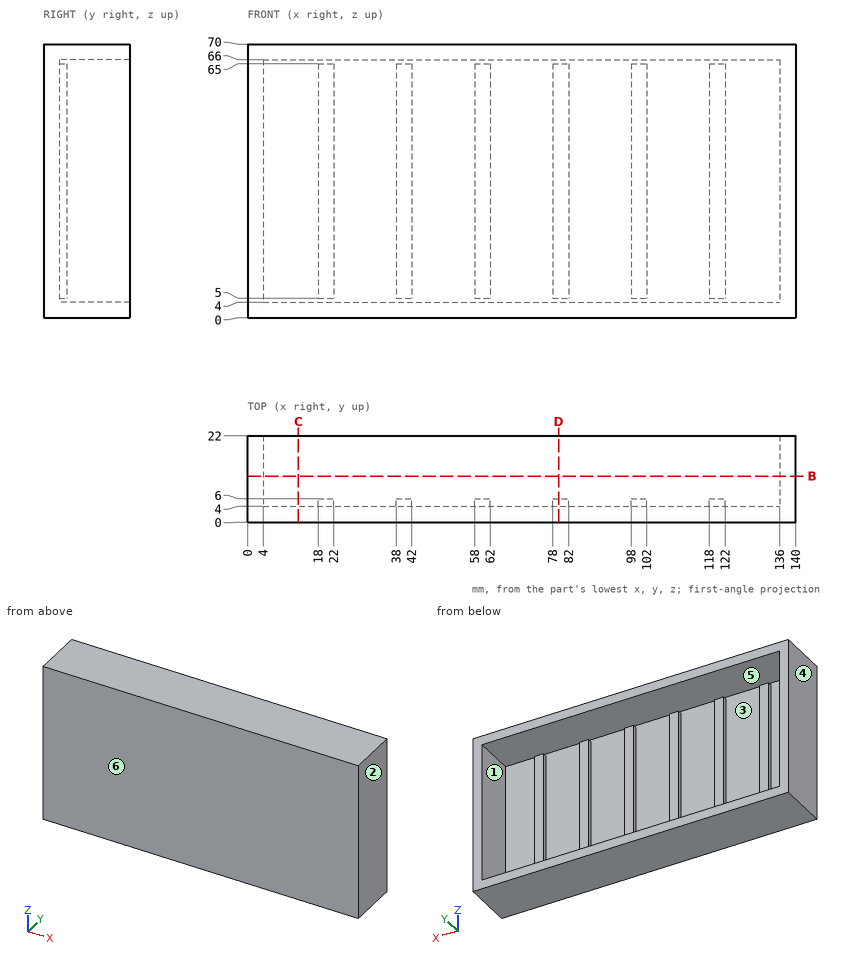
The drawing under review shows one solid part. Ordinate dimensions are in mm from its lowest x, y, z. A direction names the side the tool comes from. Coordinates: 2 decimals unless noted, no trailing zeros. Order: outer loops, then holes, each group sorted by start corner. A loop starts at its lowest first (then second) coordinate and runs counter-clockwise, first axis right, second up. Notation, with made-up numbers: (74, -19) -> (91, -19) arc R17 ccw to (91, -2) -> close; hole circle Ø1 at (14, 33.5). An arc over 180 degrees is marked (long way). One line per item, written item: value.
1) We need section C-C, the plane x = 13. Give the boundary of the cut face in (y, z), then the cut area to 3 significant figures.
Output values:
outline: (0, 0) -> (22, 0) -> (22, 4) -> (4, 4) -> (4, 66) -> (22, 66) -> (22, 70) -> (0, 70) -> close
area: 424 mm2
2) Draft analysis for pull direction X (two halves, no side actions). For the marked faces 3, 4, 5 and 6, state which applies: +X half, -X half, draft (parallel to the pull), parting line (faces both ways), or undercut.
Output values:
face 3: undercut
face 4: -X half
face 5: undercut
face 6: draft
3) We need section B-B, the plane y = 11.75. Give the boundary of the cut face in (x, z), then the cut area to 3 significant figures.
Output values:
outline: (0, 0) -> (140, 0) -> (140, 70) -> (0, 70) -> close; hole (4, 4) -> (136, 4) -> (136, 66) -> (4, 66) -> close
area: 1,620 mm2
4) To check wall thickness, follow probe 1 along X at (y, z) = (14.5, 24.5); probe 2 along Z at (x, y) = (33.5, 4.75); probe 3 along Z at (x, y) = (19.5, 5.25). State the ranges of each line that lie inside material, in increasing order. Write a range as [from, to].
Output values:
probe 1: x = [0, 4], [136, 140]
probe 2: z = [0, 4], [66, 70]
probe 3: z = [0, 4], [5, 65], [66, 70]
5) Machinability: for the marked faces 1 and 2, which of the approach directions +Z, -Z, +X, -X, +Y, -Y give a long, thin tool a straight path to every point of the face, cutting with its end or side? Answer none if there is none.
Output values:
face 1: +Y
face 2: +Z, -Z, +X, +Y, -Y
6) Clearance check with flat-ended pins moving along their axes: P1, Ø1.2, axis at x = 60, z = 36, coming from the +Y side; P2, Ø1, axis at x = 70, z = 27.5, coming from the +Y side. State where each tip first meets the part, or that it passes through.
Output values:
P1: stops at y = 6
P2: stops at y = 4
7) We need section D-D, the plane x = 79.5. Give the boundary of the cut face in (y, z), then the cut area to 3 significant figures.
Output values:
outline: (0, 0) -> (22, 0) -> (22, 4) -> (4, 4) -> (4, 5) -> (6, 5) -> (6, 65) -> (4, 65) -> (4, 66) -> (22, 66) -> (22, 70) -> (0, 70) -> close
area: 544 mm2
